```python
from build123d import *

# Parameters (mm, degrees)
F1_DEPTH = 0.8


with BuildPart() as f1:
    # F0 (on Front) → F1 (new body)
    with BuildSketch(Plane.XZ):
        with BuildLine():
            Line((0, -18.353604), (0, 36.646396))
            Line((0, 36.646396), (-12.5, 36.646396))
            Line((-12.5, 36.646396), (-12.5, -17.353604))
            ThreePointArc((-12.5, -17.353604), (-12.207107, -18.060711), (-11.5, -18.353604))
            Line((-11.5, -18.353604), (0, -18.353604))
        make_face()
        with BuildLine():
            Line((-12.5, 36.646396), (0, 36.646396))
            Line((0, 36.646396), (12.5, 36.646396))
            Line((12.5, 36.646396), (13.469037, 36.789905))
            ThreePointArc((13.469037, 36.789905), (6.839549, 38.576322), (0, 39.177953))
            ThreePointArc((0, 39.177953), (-6.839549, 38.576322), (-13.469037, 36.789905))
            Line((-13.469037, 36.789905), (-12.5, 36.646396))
        make_face()
        with BuildLine():
            Line((12.5, 36.646396), (0, 36.646396))
            Line((0, 36.646396), (0, -18.353604))
            Line((0, -18.353604), (11.5, -18.353604))
            ThreePointArc((11.5, -18.353604), (12.207107, -18.060711), (12.5, -17.353604))
            Line((12.5, -17.353604), (12.5, 36.646396))
        make_face()
    extrude(amount=F1_DEPTH)


solid = f1.part
```
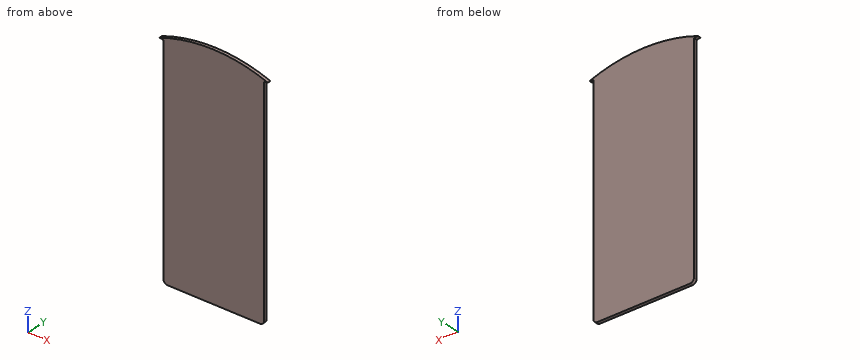
Can you work these out from the model? Positions are in its coordinate system, mm. Give positions to 0.01 mm unless a question says otherwise; leave off trailing zeros. Write each loop counter-clockwise with the first axis right and the second up, starting at its lowest first coordinate (ties: lowest second). Pieces come first, ordered by that corner, then holes. Notation, with made-up numbers: (22, -16) -> (77, -16) arc R25 ccw to (77, 7) -> close; hole circle Ø6 at (-38, 3.5). An arc over 180 degrees is marked (long way). One line per item, written item: value.
Q1. Imagine slicing it at B-B on z = -5. Please give me the cut outline in (x, y).
Results found:
outline: (-12.5, -0.8) -> (12.5, -0.8) -> (12.5, 0) -> (-12.5, 0) -> close
Q2. Imagine slicing it at C-C on x = 8.75. Please give me the cut outline in (y, z), and give its area (3 significant figures).
Results found:
outline: (-0.8, -18.35) -> (0, -18.35) -> (0, 38.19) -> (-0.8, 38.19) -> close
area: 45.2 mm^2
Q3. For P1, Ø5, axis at x = 5, z = 14.5, coming from the +Y side, with a flat end and sliding along its axis, tell me the tip position at first contact or that it passes through.
Results found:
P1: stops at y = 0
Q4. Please list where these lines run through material, in increasing order: line 1 (X direction, y = -0.2, z = -7.5); line 2 (Z direction, x = 6, y = -0.35); line 3 (Z direction, x = 4.75, y = -0.3). Write a range as [from, to].
Results found:
line 1: x = [-12.5, 12.5]
line 2: z = [-18.35, 38.72]
line 3: z = [-18.35, 38.89]
Q5. Imagine slicing it at A-A on y = -0.65. Please give me the cut outline in (x, z).
Results found:
outline: (-13.47, 36.79) -> (-12.5, 36.65) -> (-12.5, -17.35) arc R1 ccw to (-11.5, -18.35) -> (11.5, -18.35) arc R1 ccw to (12.5, -17.35) -> (12.5, 36.65) -> (13.47, 36.79) arc R39.18 ccw to (0, 39.18) arc R39.18 ccw to start
